Here's how the part is built. I have some questions about the finished solid (model axes, mm). Face numbers are marked on the shaded views. Coordinates: 2 decimals unless noted, no trailing zeros. Write each loop counter-clockwise with the first axis right and the second up, starting at its lowest first coordinate (ties: lowest second). Pieces come first, ordered by that corner, then holes. Notation, with made-up numbers: (52, -23) - (80, -23) arc R22 ccw to (80, 16) - close; hole circle Ø7 at (0.5, 64). An arc over 180 degrees is marked (long way). Answer in a Markdown table with one row per item. Add a question column.
Item 1: Imagine slicing it at C-C (y = -27). Please give me the cut outline in (x, z), plus the area to 3 significant figures.
Item 2: I'm going to push flat-ended pins straight in: pin 1 (4.5 mm diameter, centred on x = 27.5, y = -27, fed in from +Z); pin 2 (8 mm diameter, centred on x = -14.5, y = 17.5, fed in from +Z); pin 3 (5 mm diameter, centred on x = 5, z = 8, fed in from -Y); pin 4 (3 mm diameter, centred on x = 27, y = -27, fed in from +Z). Where does each tip first touch, or does it pass through?
Item 3: Imagine slicing it at D-D (y = 0). Please give me the cut outline in (x, z), plus the area to 3 significant figures.
Item 4: If I drill on probe 1 along Y at (x, z) = (-27, -4); probe 2 along Z at (x, y) = (-4.5, -6); probe 3 along Z at (x, y) = (-15.5, -21), over which ranges is the centre line in solid material (lowest first)? Write a range as from..to.
Item 5: Imagine slicing it at A-A (z = 1). State how many separate pieces and enclosed holes the cut face has, plus the area to 3 significant figures.
Item 6: Imagine slicing it at B-B (x = -27). Please give me the cut outline in (y, z), plus the area to 3 significant figures.
Item 7: We'd pull the mould along Y, two halves only. Please class the marked faces 1, 2 and 3: +Y half, -Y half, draft (parallel to the pull), parting line (faces both ways), or undercut.
from build123d import *

# Parameters (mm, degrees)
SKETCH_W     = 63.1
SKETCH_H     = 62
PAD_DEPTH    = 24
SKETCH001_R  = 24
PAD001_DEPTH = 3.2
SKETCH002_R  = 4
PAD002_DEPTH = 30
SKETCH003_R  = 2.75
PAD003_DEPTH = 2
SKETCH004_R  = 1.7
HOLE_DEPTH   = 26.001


with BuildPart() as part:
    # Sketch → Pad (new body)
    with BuildSketch(Plane.XY):
        Rectangle(SKETCH_W, SKETCH_H)
    extrude(amount=-PAD_DEPTH)

    # Sketch001 (on Face5 of Pad) → Pad001 (join)
    with BuildSketch(Plane.XY):
        Circle(SKETCH001_R)
    extrude(amount=PAD001_DEPTH)

    # Sketch002 (on Face8 of Pad001) → Pad002 (join)
    with BuildSketch(Plane.XY.offset(3.2)):
        Circle(SKETCH002_R)
    extrude(amount=PAD002_DEPTH)

    # Sketch003 (on Face4 of Pad002) → Pad003 (join)
    with BuildSketch(Plane.XY):
        with Locations((-27, 27)):
            Circle(SKETCH003_R)
        with Locations((27, 27)):
            Circle(SKETCH003_R)
        with Locations((-27, -27)):
            Circle(SKETCH003_R)
        with Locations((27, -27)):
            Circle(SKETCH003_R)
    extrude(amount=PAD003_DEPTH)

    # Sketch004 (on Face13 of Pad003) → Hole (cut, through all)
    with BuildSketch(Plane.XY.offset(2)):
        with Locations((-27, 27)):
            Circle(SKETCH004_R)
        with Locations((27, 27)):
            Circle(SKETCH004_R)
        with Locations((27, -27)):
            Circle(SKETCH004_R)
        with Locations((-27, -27)):
            Circle(SKETCH004_R)
    extrude(amount=-HOLE_DEPTH, mode=Mode.SUBTRACT)


solid = part.part
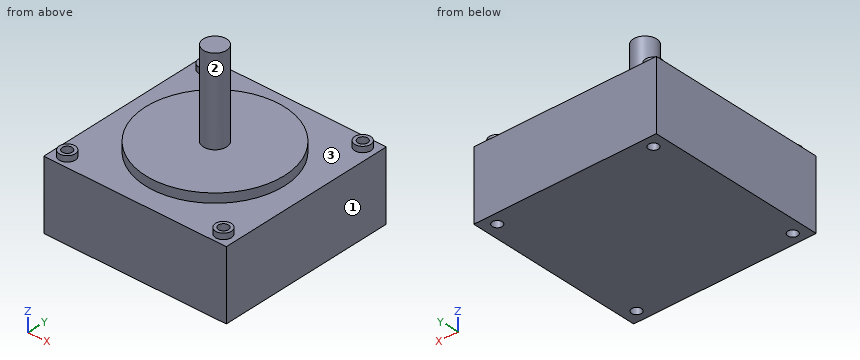
Here are the results:
| question | item | result |
|---|---|---|
| 1 | outline | (-31.55, -24) - (-28.7, -24) - (-28.7, 2) - (-29.75, 2) - (-29.75, 0) - (-31.55, 0) - close; (-25.3, -24) - (25.3, -24) - (25.3, 2) - (24.25, 2) - (24.25, 0) - (-24.25, 0) - (-24.25, 2) - (-25.3, 2) - close; (28.7, -24) - (31.55, -24) - (31.55, 0) - (29.75, 0) - (29.75, 2) - (28.7, 2) - close |
| 1 | area | 1,360 mm2 |
| 2 | pin 1 | stops at z = 2 |
| 2 | pin 2 | stops at z = 3.2 |
| 2 | pin 3 | stops at y = -3.12 |
| 2 | pin 4 | passes through |
| 3 | outline | (-31.55, -24) - (31.55, -24) - (31.55, 0) - (24, 0) - (24, 3.2) - (4, 3.2) - (4, 33.2) - (-4, 33.2) - (-4, 3.2) - (-24, 3.2) - (-24, 0) - (-31.55, 0) - close |
| 3 | area | 1,910 mm2 |
| 4 | probe 1 | y = -31..-28.7, -25.3..25.3, 28.7..31 |
| 4 | probe 2 | z = -24..3.2 |
| 4 | probe 3 | z = -24..0 |
| 5 | separate pieces | 5 |
| 5 | enclosed holes | 4 |
| 5 | area | 1,870 mm2 |
| 6 | outline | (-31, -24) - (-28.7, -24) - (-28.7, 2) - (-29.75, 2) - (-29.75, 0) - (-31, 0) - close; (-25.3, -24) - (25.3, -24) - (25.3, 2) - (24.25, 2) - (24.25, 0) - (-24.25, 0) - (-24.25, 2) - (-25.3, 2) - close; (28.7, -24) - (31, -24) - (31, 0) - (29.75, 0) - (29.75, 2) - (28.7, 2) - close |
| 6 | area | 1,330 mm2 |
| 7 | face 1 | draft |
| 7 | face 2 | parting line |
| 7 | face 3 | undercut |
